Read the model definition and answer for the solid it produces. Units are mm, in the model's axes. Face numbers are marked on the shaded views. A direction names the side the tool comes from. Give positions to 0.01 mm unless a question says otherwise; leave off trailing zeros. Order: outer loops, then holes, each group sorted by start corner. A loop starts at its lowest first (then second) coordinate and runs counter-clockwise, first axis right, second up. Notation, with made-up numbers: (75.25, 84.5) -> (84.25, 84.5) arc R21 ccw to (84.25, 90.5) -> close; hole circle Ø3 at (60, 36). An arc over 180 degrees is marked (long way). Use one line per item in the form item = value.
```python
from build123d import *

# Parameters (mm, degrees)
SKETCH1_W           = 51
SKETCH1_H           = 17
SKETCH1_R           = 2.5
BOSS_EXTRUDE1_DEPTH = 17
SKETCH6_OUTSIDE_W   = 64.276
SKETCH6_OUTSIDE_H   = 30.276
SKETCH6_OUTSIDE_W_2 = 51
SKETCH6_OUTSIDE_H_2 = 17
SKETCH6_OUTSIDE_R   = 2.5
CUT_EXTRUDE10_DEPTH = 18
SKETCH7_OUTSIDE_W   = 30.276
SKETCH7_OUTSIDE_H   = 30.276
SKETCH7_OUTSIDE_W_2 = 17
SKETCH7_OUTSIDE_H_2 = 17
CUT_EXTRUDE11_DEPTH = 17
SKETCH9_OUTSIDE_W   = 30.276
SKETCH9_OUTSIDE_H   = 30.276
SKETCH9_OUTSIDE_W_2 = 17
SKETCH9_OUTSIDE_H_2 = 17
CUT_EXTRUDE12_DEPTH = 17


with BuildPart() as part:
    # sketch1 → Boss-Extrude1 (new body)
    with BuildSketch(Plane(origin=(0, 0, 0), x_dir=(1, 0, 0), z_dir=(0, 1, 0))):
        with Locations((25.5, -8.5)):
            Rectangle(SKETCH1_W, SKETCH1_H)
        with Locations((8.5, -8.5)):
            Circle(SKETCH1_R, mode=Mode.SUBTRACT)
        with Locations((25.5, -8.5)):
            Circle(SKETCH1_R, mode=Mode.SUBTRACT)
        with Locations((42.5, -8.5)):
            Circle(SKETCH1_R, mode=Mode.SUBTRACT)
    extrude(amount=BOSS_EXTRUDE1_DEPTH)

    # Sketch6 outside → Cut-Extrude10 (cut, through all)
    with BuildSketch(Plane(origin=(0, 0, 0), x_dir=(-1, 0, 0), z_dir=(0, 0, -1))):
        with Locations((-25.5, 8.5)):
            Rectangle(SKETCH6_OUTSIDE_W, SKETCH6_OUTSIDE_H)
        with Locations((-25.5, 8.5)):
            Rectangle(SKETCH6_OUTSIDE_W_2, SKETCH6_OUTSIDE_H_2, mode=Mode.SUBTRACT)
        with Locations((-42.5, 8.5)):
            Circle(SKETCH6_OUTSIDE_R)
        with Locations((-25.5, 8.5)):
            Circle(SKETCH6_OUTSIDE_R)
        with Locations((-8.5, 8.5)):
            Circle(SKETCH6_OUTSIDE_R)
    extrude(amount=-CUT_EXTRUDE10_DEPTH, mode=Mode.SUBTRACT)

    # Sketch7 outside → Cut-Extrude11 (cut)
    with BuildSketch(Plane(origin=(51, 0, 0), x_dir=(0, 0, -1), z_dir=(1, 0, 0))):
        with Locations((-8.5, 8.5)):
            Rectangle(SKETCH7_OUTSIDE_W, SKETCH7_OUTSIDE_H)
        with Locations((-8.5, 8.5)):
            Rectangle(SKETCH7_OUTSIDE_W_2, SKETCH7_OUTSIDE_H_2, mode=Mode.SUBTRACT)
        Polygon((-8.5, 13.47803174), (-3.52196826, 8.5), (-8.5, 3.52196826), (-13.47803174, 8.5), align=None)
    extrude(amount=-CUT_EXTRUDE11_DEPTH, mode=Mode.SUBTRACT)

    # Sketch9 outside → Cut-Extrude12 (cut)
    with BuildSketch(Plane.ZY):
        with Locations((8.5, 8.5)):
            Rectangle(SKETCH9_OUTSIDE_W, SKETCH9_OUTSIDE_H)
        with Locations((8.5, 8.5)):
            Rectangle(SKETCH9_OUTSIDE_W_2, SKETCH9_OUTSIDE_H_2, mode=Mode.SUBTRACT)
        Polygon((8.5, 13.47803174), (3.52196826, 8.5), (8.5, 3.52196826), (13.47803174, 8.5), align=None)
    extrude(amount=-CUT_EXTRUDE12_DEPTH, mode=Mode.SUBTRACT)


solid = part.part
```
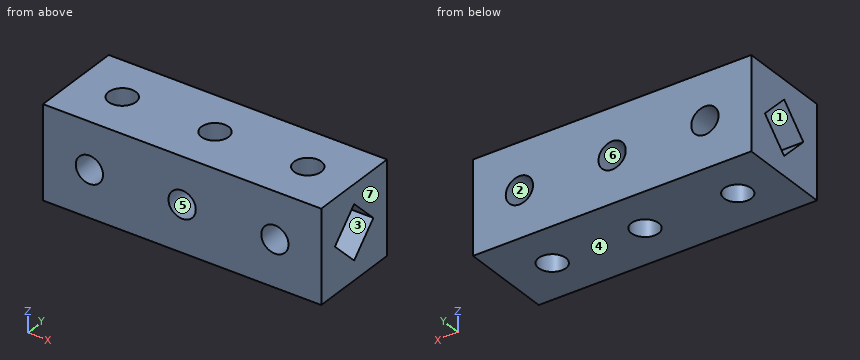
Item 1: Determine the mould class of the marked faces 4, 5, 6 and 7 for opening direction Z: +Z half, -Z half, draft (parallel to the pull), parting line (faces both ways), or undercut.
Checks:
face_4 = -Z half
face_5 = undercut
face_6 = undercut
face_7 = draft
Item 2: Given pin 1 Ø3 at (y, z) = (7.5, 10) entering from +X; pin 2 Ø4.5 at (x, z) = (8.5, 8.5) entering from -Y, each flat-ended and moving along its own axis, determine where each tip first touches the part or whether it passes through.
Checks:
pin_1 = 34
pin_2 = through
Item 3: The part is cut by section B-B on z = 15.5. Give the vertices of the cut face in (x, y), and give its area (3 significant figures).
Checks:
outline = (0, 0) -> (51, 0) -> (51, 17) -> (0, 17) -> close; hole circle Ø5 at (8.5, 8.5); hole circle Ø5 at (25.5, 8.5); hole circle Ø5 at (42.5, 8.5)
area = 808 mm²
Item 4: The part is cut by section C-C on x = 12. Give the vertices of the cut face in (y, z).
Checks:
outline = (0, 0) -> (17, 0) -> (17, 17) -> (0, 17) -> close; hole (3.52, 8.5) -> (8.5, 3.52) -> (13.48, 8.5) -> (8.5, 13.48) -> close
Item 5: Straight lines are drawn through the part: L1, parallel to X at y = 8.5, z = 2; L2, parallel to X at y = 8.5, z = 4.75; L3, parallel to X at y = 10, z = 1.5. For each, find the intervals that lie inside material, in ascending order. Write a range as from..to.
Checks:
L1 = 0..6, 11..23, 28..40, 45..51
L2 = 17..23, 28..34
L3 = 0..6.5, 10.5..23.5, 27.5..40.5, 44.5..51
Item 6: Which of the six approach directions +Z, -Z, +X, -X, +Y, -Y give full straight-line access (tool end or side, diameter ignored) to the marked faces 1, 2 and 3?
Checks:
face_1 = -X
face_2 = +Y, -Y
face_3 = +X
Item 7: The part is cut by section A-A on x = 25.5. Give the vertices of the cut face in (y, z).
Checks:
outline = (0, 0) -> (6, 0) -> (6, 6) -> (0, 6) -> close; (0, 11) -> (6, 11) -> (6, 17) -> (0, 17) -> close; (11, 0) -> (17, 0) -> (17, 6) -> (11, 6) -> close; (11, 11) -> (17, 11) -> (17, 17) -> (11, 17) -> close
Item 8: The part is cut by section D-D on z = 4.25. Give the vertices of the cut face in (x, y), and give its area (3 significant figures).
Checks:
outline = (0, 0) -> (51, 0) -> (51, 7.77) -> (44.89, 7.77) arc R2.5 cw to (40.11, 7.77) -> (34, 7.77) -> (34, 9.23) -> (40.11, 9.23) arc R2.5 cw to (44.89, 9.23) -> (51, 9.23) -> (51, 17) -> (0, 17) -> (0, 9.23) -> (6.11, 9.23) arc R2.5 cw to (10.89, 9.23) -> (17, 9.23) -> (17, 7.77) -> (10.89, 7.77) arc R2.5 cw to (6.11, 7.77) -> (0, 7.77) -> close; hole circle Ø5 at (25.5, 8.5)
area = 773 mm²
